Autodesk Inventor part; units mm, degrees
ref_plane "YZ Plane" through (0, 0, 0) normal (1, 0, 0) x (0, 1, 0)
ref_plane "XZ Plane" through (0, 0, 0) normal (0, 1, 0) x (-1, 0, 0)
ref_plane "XY Plane" through (0, 0, 0) normal (0, 0, 1) x (1, 0, 0)
sketch "Sketch1" plane through (0, 0, 0) normal (1, 0, 0) x (0, 1, 0)
  circle A0 centre (0, 0) radius 20.5
  circle A1 centre (0, 0) radius 15 construction
  line L0 (0, 0) -> (16.0369, -27.7767) construction
  line L1 (16.0369, -27.7767) -> (16.0369, 0) construction
  line L2 (16.0369, 0) -> (0, 0) construction
  circle A2 centre (0, 0) radius 14.25 construction
  line L3 (0, 0) -> (-15.2425, -26.4009) construction
  line L4 (-15.2425, -26.4009) -> (-20.5, 0) construction
  line L5 (0, 0) -> (-20.5, 0) construction
  circle A3 centre (7.5, -12.9904) radius 2
  circle A4 centre (7.5, 12.9904) radius 2
  circle A5 centre (-15, 0) radius 2
  circle A6 centre (14.25, 0) radius 2
  circle A7 centre (-7.125, 12.3409) radius 2
  circle A8 centre (-7.125, -12.3409) radius 2
  dimension "d0" = 41
  dimension "d1" = 30
  dimension "d16" = 28.5
  dimension "d15" = 60
  dimension "d22" = 60
  dimension "d28" = 4
  dimension "d31" = 360
  dimension "d33" = 4
  dimension "d36" = 360
extrude "Extrusion1" add sketch "Sketch1" along normal blind 6
chamfer "Chamfer2" distance 0.5 angle 45 1 edges at (0, -20.5, 0)
chamfer "Chamfer3" distance 2 angle 45 3 edges at (6, 5.5, 12.9904) (6, 5.5, -12.9904) (6, -17, 0)
sketch "Sketch5" plane through (6, 0, 0) normal (1, 0, 0) x (0, 0, -1)
  circle A0 centre (0, 0) radius 8.25 construction
  line L0 (0, 0) -> (16.9526, 0) construction
  line L1 (0, 0) -> (12.1845, 21.1041) construction
  circle A1 centre (4.125, 7.1447) radius 2
  circle A2 centre (-8.25, 0) radius 2
  circle A3 centre (4.125, -7.1447) radius 2
  dimension "d44" = 16.5
  dimension "d45" = 60
  dimension "d46" = 4
  dimension "d49" = 360
extrude "Extrusion3" cut sketch "Sketch5" against normal blind 3
properties part number "ab_hip_joint_connector"
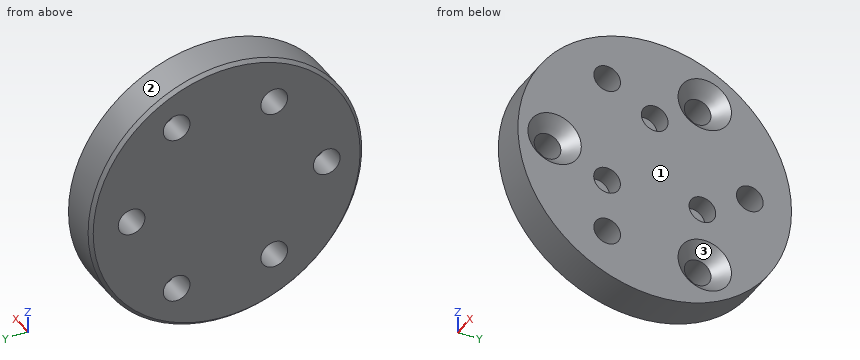
CAD build for the part. Positions are in the model's coordinates, mm. Face numbers are marked on the shaded views. Round coordinates to 2 decimals unless told otherwise and drop trailing zeros. Loops run counter-clockwise (first coordinate to the right, second up) from the corner with the lowest first, then second, coordinate; pieces in that order, holes last. Notation, with made-up numbers: M 58.25,-26 L 69.25,-26 A20 cw 69.25,-16 Z; hole C -38.75,67.5 d3. An arc over 180 degrees is marked long. Return JSON: item names as keys, results as strings. Group by question number.
(1) Saw through at C-C, the plane x = 1.15. List the corners of the cut face in (y, z) (3 decimals).
(2) Saw through at A-A, the plane z = 0. List the corners of the cut face in (x, y).
(3) Wall check: probe 1 along Y at (x, z) = (2.35, -0.5); probe 2 along Z at (x, y) = (1.3, 7.5); probe 3 along Y at (x, z) = (1.1, 13.5). Give the ranges that are in metal, low to high. Write a range as [from, to].
(4) Saw through at D-D, the plane x = 5.25. Give the number of separate pieces and of enclosed holes in the cut face, and give its area (3 significant figures).
(5) Mould opens along Z. For the marked faces 1, 2 and 3 say: +Z half, -Z half, draft (parallel to the pull), parting line (faces both ways), or undercut.
(6) Drop flat-ended pins along their axis: P1, Ø1, axis at x = 3.5, z = -12.5, coming from the -Y side; P2, Ø1.2, axis at y = 0, z = 9, coming from the +X side; P3, Ø2, axis at x = 1.5, y = -11.5, coming from the +Z side; P4, Ø2.5, axis at y = -7.12, z = -12.34, coming from the +X side. Give the stop position or say it passes through.
(7) Saw through at B-B, the plane y = 0. List the corners of the cut face in (x, z), and give its area (3 significant figures).
Answer list:
{
 "1": {"outline": "C 0,0 d41; hole C -15,0 d4; hole C -7.125,-12.341 d4; hole C -7.125,12.341 d4; hole C 7.5,-12.99 d4; hole C 7.5,12.99 d4; hole C 14.25,0 d4"},
 "2": {"outline": "M 0,-20 L 0.5,-20.5 L 6,-20.5 L 6,-19 L 4,-17 L 0,-17 Z; M 0,-13 L 4,-13 L 6,-11 L 6,12.25 L 0,12.25 Z; M 0,16.25 L 6,16.25 L 6,20.5 L 0.5,20.5 L 0,20 Z"},
 "3": {"probe 1": "[-20.49, -16.94], [-13.06, 12.31], [16.19, 20.49]", "probe 2": "[-19.08, -14.99], [-10.99, 10.99], [14.99, 19.08]", "probe 3": "[-15.43, -8.75], [-5.5, 5.57], [9.43, 15.43]"},
 "4": {"separate pieces": "1", "enclosed holes": "9", "area": "1,150 mm2"},
 "5": {"face 1": "draft", "face 2": "parting line", "face 3": "undercut"},
 "6": {"P1": "y = -16.62", "P2": "x = 3", "P3": "z = 17.61", "P4": "through"},
 "7": {"outline": "M 0,-20 L 0.5,-20.5 L 6,-20.5 L 6,6.25 L 3,6.25 L 3,10.25 L 6,10.25 L 6,20.5 L 0.5,20.5 L 0,20 Z", "area": "234 mm2"}
}
